For this review, take the finished solid that the model builds, in its own axes (mm). Give positions to 0.01 mm unless a question says otherwise; leave off trailing zeros. Order: outer loops, then holes, each group sorted by start corner. A loop starts at its lowest first (then second) coordinate and runs counter-clockwise, first axis right, second up.
Item 1: For P1, Ø1.5, axis at x = -15.5, y = 0, coming from the +Z side; P2, Ø3, axis at x = 21, y = 2.5, coming from the +Z side (3 decimals), all flat-tipped, find the tip position at first contact; note any pin that passes through.
Item 2: Consider section B-B (z = -10). Give the boundary of the cut face in (x, y) (3 decimals).
Item 3: Consider section C-C (x = 18.5). Give the boundary of the cut face in (y, z) (3 decimals).
Item 4: Consider section D-D (x = 74). Give the boundary of the cut face in (y, z) (3 decimals), plus the area to 3 significant figures.
Item 5: For probe 1 along Z at (x, y) = (-40, 1); probe 2 along X at (y, z) = (-2.5, 73.5); probe 3 along X at (y, z) = (2.5, 75), list the stretches that pass through material, from the lowest coordinate up.
Item 6: Consider section A-A (y = -1.5). Give the boundary of the cut face in (x, z) (3 decimals), plus the area to 3 significant figures.
```python
from build123d import *

# Parameters (mm, degrees)
F0_R     = 50.8
F1_DEPTH = 3.175


with BuildPart() as f1:
    # F0 (on Front) → F1 (new body, symmetric)
    with BuildSketch(Plane.XZ):
        with BuildLine():
            ThreePointArc((0, 88.9), (-62.861793, -62.861793), (88.9, 0))
            ThreePointArc((88.9, 0), (62.861793, 62.861793), (0, 88.9))
        make_face()
        Circle(F0_R, mode=Mode.SUBTRACT)
        with BuildLine():
            ThreePointArc((5.1562, 73.025), (-3.645984, 69.379016), (0, 78.1812))
            ThreePointArc((0, 78.1812), (3.645984, 76.670984), (5.1562, 73.025))
        make_face(mode=Mode.SUBTRACT)
    extrude(amount=F1_DEPTH, both=True)


solid = f1.part
```
Resolved:
1. P1: stops at z = 87.67
1. P2: stops at z = 86.735
2. outline: (-88.336, -3.175) - (-49.806, -3.175) - (-49.806, 3.175) - (-88.336, 3.175) - close; (49.806, -3.175) - (88.336, -3.175) - (88.336, 3.175) - (49.806, 3.175) - close
3. outline: (-3.175, -86.954) - (3.175, -86.954) - (3.175, -47.312) - (-3.175, -47.312) - close; (-3.175, 47.312) - (3.175, 47.312) - (3.175, 86.954) - (-3.175, 86.954) - close
4. outline: (-3.175, -49.267) - (3.175, -49.267) - (3.175, 49.267) - (-3.175, 49.267) - close
4. area: 626 mm2
5. probe 1: z = -79.39 to -31.32, 31.32 to 79.39
5. probe 2: x = -50.01 to -5.13, 5.13 to 50.01
5. probe 3: x = -47.73 to -4.76, 4.76 to 47.73
6. outline: circle Ø177.8 at (0, 0); hole circle Ø101.6 at (0, 0); hole circle Ø10.312 at (0, 73.025)
6. area: 16,600 mm2
